Can you work these out from the model? Positions are in its coordinate system, mm. A direction names the side the tool comes from. Coordinates: 2 decimals unless noted, no trailing zeros. Use one line per item in the form item = value. Start each with the question number.
```python
from build123d import *

# Parameters (mm, degrees)
SKETCH_1_W      = 180
SKETCH_1_H      = 227
SKETCH_1_R      = 1.625
EXTRUDE_1_DEPTH = 2


with BuildPart() as part:
    # 草图1 → 凸台-拉伸1 (new body)
    with BuildSketch(Plane.XY):
        Rectangle(SKETCH_1_W, SKETCH_1_H)
        with Locations((-15, 88.5)):
            Circle(SKETCH_1_R, mode=Mode.SUBTRACT)
        with Locations((55, 88.5)):
            Circle(SKETCH_1_R, mode=Mode.SUBTRACT)
        with Locations((55, 18.5)):
            Circle(SKETCH_1_R, mode=Mode.SUBTRACT)
        with Locations((-15, 18.5)):
            Circle(SKETCH_1_R, mode=Mode.SUBTRACT)
        with Locations((-80, 103.5)):
            Circle(SKETCH_1_R, mode=Mode.SUBTRACT)
        with Locations((0, 103.5)):
            Circle(SKETCH_1_R, mode=Mode.SUBTRACT)
        with Locations((80, 103.5)):
            Circle(SKETCH_1_R, mode=Mode.SUBTRACT)
        with Locations((80, -103.5)):
            Circle(SKETCH_1_R, mode=Mode.SUBTRACT)
        with Locations((0, -103.5)):
            Circle(SKETCH_1_R, mode=Mode.SUBTRACT)
        with Locations((-80, -103.5)):
            Circle(SKETCH_1_R, mode=Mode.SUBTRACT)
        with Locations((80, 0)):
            Circle(SKETCH_1_R, mode=Mode.SUBTRACT)
        with Locations((-80, 0)):
            Circle(SKETCH_1_R, mode=Mode.SUBTRACT)
        with BuildLine():
            Line((63.076132364, 88.90914901), (52.469530647, 99.515750728))
            ThreePointArc((52.469530647, 99.515750728), (52.469530647, 108.001032102), (60.954812021, 108.001032102))
            Line((60.954812021, 108.001032102), (71.561413739, 97.394430384))
            ThreePointArc((71.561413739, 97.394430384), (71.561413739, 88.90914901), (63.076132364, 88.90914901))
        make_face(mode=Mode.SUBTRACT)
    extrude(amount=EXTRUDE_1_DEPTH)


solid = part.part
```
1) Which directions (+Z, -Z, +X, -X, +Y, -Y) give clear straight access to the entire face, cutting with the end or side of a thin tool? Please do faces 1 (the face through (66.184, 102.772, 0.986)), 2 (the face through (-1, 2, 2)).
2) Please list where these lines run through material, in increasing order: line 1 (Y direction, x = -80, z = 0.75) (3 decimals); line 2 (X direction, y = -103.5, z = 0.55) (3 decimals); line 3 (Y direction, x = -15, z = 0.9) (3 decimals).
3) If we mould it in two halves opening along Y, with no side actions, what happens to faces 3 (the face through (57.847, 94.138, 0.986)), 4 (the face through (-1, 2, 0))? For each: +Y half, -Y half, draft (parallel to the pull), parting line (faces both ways), or undercut.
Computed values:
q1.face_1 = +Z, -Z
q1.face_2 = +Z, +X, -X, +Y, -Y
q2.line_1 = -113.5 to -105.125, -101.875 to -1.625, 1.625 to 101.875, 105.125 to 113.5
q2.line_2 = -90 to -81.625, -78.375 to -1.625, 1.625 to 78.375, 81.625 to 90
q2.line_3 = -113.5 to 16.875, 20.125 to 86.875, 90.125 to 113.5
q3.face_3 = undercut
q3.face_4 = draft
